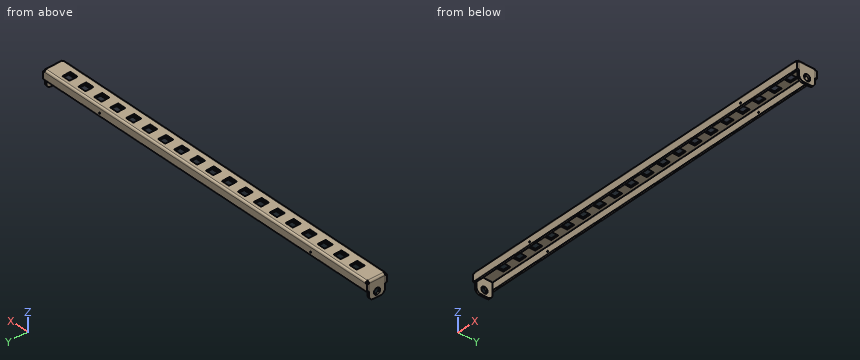
from build123d import *

# Parameters (mm, degrees)
SKETCH_1_W                         = 406.5
SKETCH_1_H                         = 22
SM_BASE_FLANGE_1_DEPTH             = 2
SM_EDGE_FLANGE_1_STRIP_W           = 8.2
SM_EDGE_FLANGE_1_STRIP_H           = 2
SM_EDGE_FLANGE_1_STRIP_CUT_DEPTH   = 406.5
SM_EDGE_FLANGE_1_STRIP_2_W         = 8.2
SM_EDGE_FLANGE_1_STRIP_2_H         = 2
SM_EDGE_FLANGE_1_STRIP_CUT_2_DEPTH = 406.5
SM_EDGE_FLANGE_1_DEPTH             = 406.5
SM_EDGE_FLANGE_1_BEND_DEPTH        = 406.5
SM_START                           = -11
SM_EDGE_FLANGE_2_DEPTH             = 22
SM_EDGE_FLANGE_2_2_DEPTH           = 2.1
SM_START_2                         = 8.9
SM_EDGE_FLANGE_2_3_DEPTH           = 2.1
SM_START_3                         = -8.9
SM_EDGE_FLANGE_2_4_DEPTH           = 17.8
SKETCH_18_W                        = 9
SKETCH_18_H                        = 9
CUT_EXTRUDE_1_DEPTH                = 10
PATTERN_LINEAR_1_COUNT             = 19
PATTERN_LINEAR_1_PITCH             = 20
FILLET_1_R                         = 5
SKETCH_19_R                        = 3.5
CUT_EXTRUDE_2_DEPTH                = 408.140332072
CUT_EXTRUDE_3_DEPTH                = 206.413150747
CUT_EXTRUDE_3_DEPTH_BACK           = 206.413150747
SKETCH_20_R                        = 0.75


# Read off the part's stored shape, not the designer's step: 边线-法兰2
# Sheet-metal steps are written as plain solids
with BuildPart() as part:
    # Sketch 1 → 基体-法兰1 (new body)
    with BuildSketch(Plane.XY):
        Rectangle(SKETCH_1_W, SKETCH_1_H)
    extrude(amount=-SM_BASE_FLANGE_1_DEPTH)

    # 边线-法兰1 strip (across the edge) → 边线-法兰1 strip cut (cut)
    with BuildSketch(Plane(origin=(203.25, -11, -2), x_dir=(0, 1, 0), z_dir=(-1, 0, 0))):
        with Locations((-2, -1)):
            Rectangle(SM_EDGE_FLANGE_1_STRIP_W, SM_EDGE_FLANGE_1_STRIP_H)
    extrude(amount=SM_EDGE_FLANGE_1_STRIP_CUT_DEPTH, mode=Mode.SUBTRACT)

    # 边线-法兰1 strip 2 (across the edge) → 边线-法兰1 strip cut 2 (cut)
    with BuildSketch(Plane(origin=(-203.25, 11, -2), x_dir=(0, -1, 0), z_dir=(1, 0, 0))):
        with Locations((-2, -1)):
            Rectangle(SM_EDGE_FLANGE_1_STRIP_2_W, SM_EDGE_FLANGE_1_STRIP_2_H)
    extrude(amount=SM_EDGE_FLANGE_1_STRIP_CUT_2_DEPTH, mode=Mode.SUBTRACT)

    # 边线-法兰1 section (across the edge) → 边线-法兰1 (add)
    with BuildSketch(Plane(origin=(203.25, -11, -2), x_dir=(0, 1, 0), z_dir=(-1, 0, 0))):
        with BuildLine():
            Line((0, 0.1), (0, 8))
            Line((0, 8), (2, 8))
            Line((2, 8), (2, 0.1))
            ThreePointArc((2, 0.1), (2.029289322, 0.029289322), (2.1, 0))
            Line((2.1, 0), (2.1, -2))
            ThreePointArc((2.1, -2), (0.61507576, -1.38492424), (0, 0.1))
        make_face()
    extrude(amount=SM_EDGE_FLANGE_1_DEPTH)

    # 边线-法兰1 section 2 (across the edge) → 边线-法兰1 bend (add)
    with BuildSketch(Plane(origin=(-203.25, 11, -2), x_dir=(0, -1, 0), z_dir=(1, 0, 0))):
        with BuildLine():
            Line((0, 0.1), (0, 8))
            Line((0, 8), (2, 8))
            Line((2, 8), (2, 0.1))
            ThreePointArc((2, 0.1), (2.029289322, 0.029289322), (2.1, 0))
            Line((2.1, 0), (2.1, -2))
            ThreePointArc((2.1, -2), (0.61507576, -1.38492424), (0, 0.1))
        make_face()
    extrude(amount=SM_EDGE_FLANGE_1_BEND_DEPTH)

    # 边线-法兰2 outline → 边线-法兰2 (cut)
    with BuildSketch(Plane(origin=(0, 0, 0), x_dir=(1, 0, 0), z_dir=(0, 1, 0)).offset(SM_START)):
        with BuildLine():
            Line((201.25, 2.1), (201.15, 2.1))
            Line((201.15, 2.1), (201.15, 2))
            ThreePointArc((201.15, 2), (201.220710678, 2.029289322), (201.25, 2.1))
        make_face()
        with BuildLine():
            ThreePointArc((203.25, 2.1), (202.63492424, 0.61507576), (201.15, 0))
            Line((201.15, 0), (203.25, 0))
            Line((203.25, 0), (203.25, 2.1))
        make_face()
        with BuildLine():
            ThreePointArc((-201.25, 2.1), (-201.220710678, 2.029289322), (-201.15, 2))
            Line((-201.15, 2), (-201.15, 2.1))
            Line((-201.15, 2.1), (-201.25, 2.1))
        make_face()
        with BuildLine():
            Line((-203.25, 0), (-201.15, 0))
            ThreePointArc((-201.15, 0), (-202.63492424, 0.61507576), (-203.25, 2.1))
            Line((-203.25, 2.1), (-203.25, 0))
        make_face()
    extrude(amount=SM_EDGE_FLANGE_2_DEPTH, mode=Mode.SUBTRACT)

    # Sm Edge Flange 2 2 outline → Sm Edge Flange 2 2 (cut)
    with BuildSketch(Plane(origin=(0, 0, 0), x_dir=(1, 0, 0), z_dir=(0, 1, 0)).offset(SM_START)):
        with BuildLine():
            Line((203.25, 2.1), (201.25, 2.1))
            ThreePointArc((201.25, 2.1), (201.220710678, 2.029289322), (201.15, 2))
            Line((201.15, 2), (201.15, 0))
            ThreePointArc((201.15, 0), (202.63492424, 0.61507576), (203.25, 2.1))
        make_face()
        with BuildLine():
            ThreePointArc((-203.25, 2.1), (-202.63492424, 0.61507576), (-201.15, 0))
            Line((-201.15, 0), (-201.15, 2))
            ThreePointArc((-201.15, 2), (-201.220710678, 2.029289322), (-201.25, 2.1))
            Line((-201.25, 2.1), (-203.25, 2.1))
        make_face()
    extrude(amount=SM_EDGE_FLANGE_2_2_DEPTH, mode=Mode.SUBTRACT)

    # Sm Edge Flange 2 3 outline → Sm Edge Flange 2 3 (cut)
    with BuildSketch(Plane(origin=(0, 0, 0), x_dir=(1, 0, 0), z_dir=(0, 1, 0)).offset(SM_START_2)):
        with BuildLine():
            Line((203.25, 2.1), (201.25, 2.1))
            ThreePointArc((201.25, 2.1), (201.220710678, 2.029289322), (201.15, 2))
            Line((201.15, 2), (201.15, 0))
            ThreePointArc((201.15, 0), (202.63492424, 0.61507576), (203.25, 2.1))
        make_face()
        with BuildLine():
            ThreePointArc((-203.25, 2.1), (-202.63492424, 0.61507576), (-201.15, 0))
            Line((-201.15, 0), (-201.15, 2))
            ThreePointArc((-201.15, 2), (-201.220710678, 2.029289322), (-201.25, 2.1))
            Line((-201.25, 2.1), (-203.25, 2.1))
        make_face()
    extrude(amount=SM_EDGE_FLANGE_2_3_DEPTH, mode=Mode.SUBTRACT)

    # Sm Edge Flange 2 4 outline → Sm Edge Flange 2 4 (add)
    with BuildSketch(Plane(origin=(0, 0, 0), x_dir=(1, 0, 0), z_dir=(0, 1, 0)).offset(SM_START_3)):
        with BuildLine():
            Line((201.25, 20), (201.25, 2.1))
            ThreePointArc((201.25, 2.1), (201.220710678, 2.029289322), (201.15, 2))
            Line((201.15, 2), (203.247617696, 2))
            ThreePointArc((203.247617696, 2), (203.24940434, 2.049985814), (203.25, 2.1))
            Line((203.25, 2.1), (203.25, 20))
            Line((203.25, 20), (201.25, 20))
        make_face()
        with BuildLine():
            Line((-203.247617696, 2), (-201.15, 2))
            ThreePointArc((-201.15, 2), (-201.220710678, 2.029289322), (-201.25, 2.1))
            Line((-201.25, 2.1), (-201.25, 20))
            Line((-201.25, 20), (-203.25, 20))
            Line((-203.25, 20), (-203.25, 2.1))
            ThreePointArc((-203.25, 2.1), (-203.24940434, 2.049985814), (-203.247617696, 2))
        make_face()
    extrude(amount=SM_EDGE_FLANGE_2_4_DEPTH)

    # 草图18 → 切除-拉伸1 (cut)
    with BuildSketch(Plane.XY):
        with Locations((-179.25, 1)):
            Rectangle(SKETCH_18_W, SKETCH_18_H)
    cut_extrude_1 = extrude(amount=-CUT_EXTRUDE_1_DEPTH, mode=Mode.SUBTRACT)

    # 阵列(线性)1: 切除-拉伸1 ×19
    with Locations(*[(i * PATTERN_LINEAR_1_PITCH, 0, 0) for i in range(1, PATTERN_LINEAR_1_COUNT)]):
        add(cut_extrude_1, mode=Mode.SUBTRACT)

    # 圆角1
    fillet_1_edges = [part.edges().sort_by_distance(p)[0] for p in [
        (-202.25, -8.9, -20),
        (-202.25, 8.9, -20),
        (202.25, 8.9, -20),
        (202.25, -8.9, -20),
    ]]
    fillet(fillet_1_edges, radius=FILLET_1_R)

    # 草图19 → 切除-拉伸2 (cut, through all)
    with BuildSketch(Plane(origin=(203.25, 0, 0), x_dir=(0, 0, -1), z_dir=(1, 0, 0))):
        with Locations((14, 0)):
            Circle(SKETCH_19_R)
    extrude(amount=-CUT_EXTRUDE_2_DEPTH, mode=Mode.SUBTRACT)

    # 草图20 → 切除-拉伸3 (cut, two sides: drawn at the far end of the back side and taken through both)
    with BuildSketch(Plane.XZ.offset(11).offset(-CUT_EXTRUDE_3_DEPTH_BACK)):
        with Locations(Location((132.25, -7, 0), (0, 0, 270))):
            Circle(SKETCH_20_R)
        with Locations(Location((-132.25, -7, 0), (0, 0, 270))):
            Circle(SKETCH_20_R)
    extrude(amount=CUT_EXTRUDE_3_DEPTH + CUT_EXTRUDE_3_DEPTH_BACK, mode=Mode.SUBTRACT)


solid = part.part
Work out the finished part from the listing and answer in its coordinate system (mm). Round coordinates to 2 decimals unless told otherwise and drop trailing zeros. Write each loop counter-clockwise with the first axis right and the second up, starting at its lowest first coordinate (ties: lowest second). Pieces come first, ordered by that corner, then holes.
1) A cutting plane is placed at B-B (y = 0). Give the number of separate pieces and of enclosed holes in the cut face, plus the area to 3 significant figures.
2) Straight lines are drawn through the part: line 1 (X direction, y = 9.5, z = -7); line 2 (X direction, y = -5.75, z = -13.25); line 3 (Y direction, x = 45, z = -7.5). For each, find the intervals that lie inside material, in ascending order.
3) A cutting plane is placed at A-A (x = 171). Give the vertices of the cut face in (y, z).
4) Given pin 1 Ø1 at (y, z) = (2.5, -1) entering from -X; pin 2 Ø1 at (x, y) = (29.5, -1) entering from +Z; pin 3 Ø2 at (y, z) = (1.5, -0.5) entering from +X; pin 4 Ø0.6 at (y, z) = (2, -0.5) entering from +X, each flat-ended and moving along its own axis, determine where each tip first touches the part or whether it passes through.
Completed:
1. separate pieces: 22
1. enclosed holes: 0
1. area: 513 mm2
2. line 1: x = -203.25 to -133, -131.5 to 131.5, 133 to 203.25
2. line 2: x = -203.25 to -201.25, 201.25 to 203.25
2. line 3: y = -11 to -9, 9 to 11
3. outline: (-11, -10) - (-9, -10) - (-9, -2.1) arc R0.1 cw to (-8.9, -2) - (8.9, -2) arc R0.1 cw to (9, -2.1) - (9, -10) - (11, -10) - (11, -2.1) arc R2.1 ccw to (8.9, 0) - (-8.9, 0) arc R2.1 ccw to (-11, -2.1) - close
4. pin 1: stops at x = -203.16
4. pin 2: stops at z = 0
4. pin 3: stops at x = 203.16
4. pin 4: stops at x = 202.8
